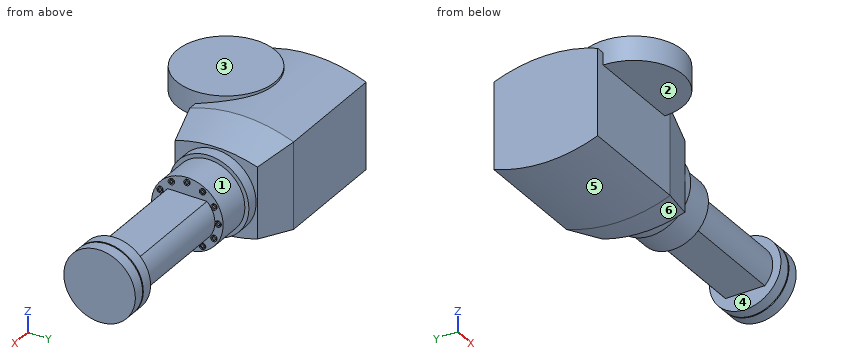
Autodesk Fusion 360 part; units mm, degrees
sketch "Sketch1" plane through (0, 0, 0) normal (1, 0, 0) x (0, 0, -1)
  line L0 (0, 0) -> (0, 45)
  line L1 (0, 0) -> (0, -45)
  line L2 (0, 45) -> (37.5, 45)
  line L3 (0, 45) -> (-37.5, 45)
  line L4 (0, -45) -> (37.5, -45)
  line L5 (0, -45) -> (-37.5, -45)
  arc A0 (-37.5, 45) -> (-37.5, -45) centre (79.119, 0) ccw
  arc A1 (37.5, -45) -> (37.5, 45) centre (-79.119, 0) ccw
  dimension "d1" = 45
  dimension "d2" = 45
  dimension "d3" = 37.5
  dimension "d4" = 37.5
  dimension "d5" = 37.5
  dimension "d6" = 37.5
  dimension "d8" = 125
extrude "Extrude1" add sketch "Sketch1" along normal blind 100
extrude "Extrude2" add 1 faces at (100, -15.2642, -14.2806) along direction (1, 0, 0) blind 35 draft -15
sketch "Sketch2" plane through (135, 0, 0) normal (1, 0, 0) x (0, 0, -1)
  line L0 (-30.8786, -35.6218) -> (30.8786, -35.6218)
  arc A0 (30.8786, -35.6218) -> (30.8786, 35.6218) centre (-79.119, 0) ccw
  line L1 (30.8786, 35.6218) -> (-30.8786, 35.6218)
  arc A1 (-30.8786, 35.6218) -> (-30.8786, -35.6218) centre (79.119, 0) ccw
  circle A2 centre (0, 0) radius 34.5
  dimension "d13" = 69
extrude "Extrude3" add sketch "Sketch2" along normal blind 10 contours A2
sketch "Sketch3" plane through (145, 0, 0) normal (1, 0, 0) x (0, 0, -1)
  circle A0 centre (0, 0) radius 34.5
  circle A1 centre (0, 0) radius 31
  dimension "d16" = 62
extrude "Extrude4" add sketch "Sketch3" along normal blind 30 contours A1
sketch "Sketch4" plane through (175, 0, 0) normal (1, 0, 0) x (0, 0, -1)
  circle A0 centre (0, 0) radius 31
  line L0 (0, 0) -> (27, 0)
  circle A1 centre (27, 0) radius 2.5
  circle A2 centre (27, 0) radius 1.5
  dimension "d19" = 27
  dimension "d20" = 5
  dimension "d21" = -1
extrude "Extrude5" add sketch "Sketch4" along normal blind 1 contours A1
pattern_circular "C-Pattern1" count 12 over 360 about axis through (175, 0, 0) along (1, 0, 0) of "Extrude5"
sketch "Sketch5" plane through (175, 0, 0) normal (1, 0, 0) x (0, 0, -1)
  circle A0 centre (27, 0) radius 2.5
  circle A1 centre (0, 0) radius 31
  circle A2 centre (23.3827, 13.5) radius 2.5
  circle A3 centre (13.5, 23.3827) radius 2.5
  circle A4 centre (0, 27) radius 2.5
  circle A5 centre (-13.5, 23.3827) radius 2.5
  circle A6 centre (-23.3827, 13.5) radius 2.5
  circle A7 centre (-27, 0) radius 2.5
  circle A8 centre (-23.3827, -13.5) radius 2.5
  circle A9 centre (-13.5, -23.3827) radius 2.5
  circle A10 centre (0, -27) radius 2.5
  circle A11 centre (13.5, -23.3827) radius 2.5
  circle A12 centre (23.3827, -13.5) radius 2.5
  line L0 (0, 0) -> (16, 0)
  line L1 (16, 0) -> (16, 17)
  line L2 (16, 0) -> (16, -17)
  line L3 (0, 0) -> (0, -8.0593)
  line L4 (-16, 0) -> (-16, 17)
  line L5 (-16, 0) -> (-16, -17)
  arc A13 (16, 17) -> (-16, 17) centre (0, 1.9003) ccw
  arc A14 (-16, -17) -> (16, -17) centre (0, -1.9003) ccw
  dimension "d26" = 16
  dimension "d27" = 17
  dimension "d28" = 17
  dimension "d29" = 22
extrude "Extrude6" add sketch "Sketch5" along normal blind 100 contours L1 L2 L4 L5 A13 A14
sketch "Sketch6" plane through (275, 0, 0) normal (1, 0, 0) x (0, 0, -1)
  line L0 (-16, 17) -> (-16, -17)
  arc A0 (-16, -17) -> (16, -17) centre (0, -1.9003) ccw
  line L1 (16, -17) -> (16, 17)
  arc A1 (16, 17) -> (-16, 17) centre (0, 1.9003) ccw
  circle A2 centre (0, 0) radius 31
  circle A3 centre (0, 0) radius 30
  dimension "d32" = 62
  dimension "d35" = -1
extrude "Extrude7" add sketch "Sketch6" along normal blind 10 contours L0 A0 L1 A1 | A2 | A3
sketch "Sketch7" plane through (285, 0, 0) normal (1, 0, 0) x (0, 0, -1)
  circle A0 centre (0, 0) radius 31
  circle A1 centre (0, 0) radius 30
  dimension "d36" = -1
extrude "Extrude8" add sketch "Sketch7" along normal blind 1 contours A1
sketch "Sketch8" plane through (286, 0, 0) normal (1, 0, 0) x (0, 0, -1)
  circle A0 centre (0, 0) radius 30
  circle A1 centre (0, 0) radius 31
  dimension "d39" = 62
extrude "Extrude9" add sketch "Sketch8" along normal blind 10 contours A0 | A1
ref_plane "WorkPlane1" through (0, 45, 37.5) normal (0, 0, 1) x (1, 0, 0)
sketch "Sketch9" plane through (0, 0, 37.5) normal (0, 0, 1) x (1, 0, 0)
  circle A0 centre (50, -45) radius 42.5
  dimension "d43" = 85
extrude "Extrude10" add sketch "Sketch9" along normal mid plane 21
equation "d44 = ( 21 / 2 ) * 1 mm"
Verification items for the finished model (mm, model axes). Face numbers are marked on the shaded views. A direction names the side the tool comes from. Give positions to 0.01 mm unless a question says otherwise; leave off trailing zeros. Loops run counter-clockwise (first coordinate to the right, second up) from the corner with the lowest first, then second, coordinate; pieces in that order, holes last. Notation, with made-up numbers: (-28, -21.5) - (-16, -21.5) arc R26 ccw to (-16, 11.5) - close; hole circle Ø3 at (66.5, 83.5). An arc over 180 degrees is marked (long way). Write item = value, one per line. Start each with the question number.
Q1. Cross-section at C-C, the plane y = -74. Enter the section's corners in (x, z).
Q2. Tool access check on the marked faces 1, 2 and 3. Record the directions out of +Z, -Z, +X, -X, +Y, -Y that give a thin tool (end or side, any length) a straight path to the whole face; none if there is none.
Q3. Cross-section at A-A, the plane x = 33.5. Enter the section's corners in (y, z).
Q4. Depth check by flat-ended pin: P1, Ø12, axis at x = 69, z = 1.5, coming from the -Y side; P2, Ø2, axis at x = 168, y = 11, coming from the +Z side; P3, Ø6, axis at x = 69, y = -37, coming from the -Z side. Enter the tip coordinate at first touch or a pass-through.
Q5. Mould release check, pull along X, two halves, no side actions. Record for the marked faces 4, 5 and 6: released by +X, released by -X, zero draft, split by the parting line, or undercut.
Q6. Thickness scan on line 1 (Y direction, x = 175.3, z = 0); line 2 (Z direction, x = 175.7, y = 0); line 3 (X direction, y = 4.5, z = 28). Record the ranges inside material, lowest first.
Answer key:
q1.outline = (18.93, 27) - (81.07, 27) - (81.07, 48) - (18.93, 48) - close
q2.face_1 = +X
q2.face_2 = -Z, +X, -X, -Y
q2.face_3 = +Z, +X, -X, +Y, -Y
q3.outline = (-84.17, 27) - (-45, 27) - (-45, -37.5) arc R125 ccw to (45, -37.5) - (45, 37.5) arc R125 ccw to (-5.83, 45.74) - (-5.83, 48) - (-84.17, 48) - close
q4.P1 = -45
q4.P2 = 29.34
q4.P3 = -41.17
q5.face_4 = undercut
q5.face_5 = zero draft
q5.face_6 = released by +X
q6.line_1 = -29.5 to -28.5, -25.5 to -24.5, -23.9 to 23.9, 24.5 to 25.5, 28.5 to 29.5
q6.line_2 = -29.5 to -28.5, -25.5 to -24.5, -16 to 16, 24.5 to 25.5, 28.5 to 29.5
q6.line_3 = 0 to 175, 275 to 296
